Check sheet for the modelled part. Datum: model origin and axes. Units: mm. A direction names the side the tool comes from. Round coordinates to 2 decimals unless told otherwise and drop trailing zeros. Write each loop counter-clockwise with the first axis right and the second up, starting at its lowest first coordinate (ties: lowest second). Pieces come first, ordered by that corner, then holes.
Item 1: Set-up check for faces 1 (the flat face through (165.207, -94, 2)), 2 (the flat face through (83, -151, 2)), 3 (the flat face through (147, -104, 5)): record each of +Z, -Z, +X, -X, +Y, -Y from which the full face is reachable in a straight line by a thin tool's end or side.
Item 2: Section check B-B, the plane y = -133. Record the cut outline in (x, z).
Item 3: Release check for a two-part mould opening along X. For faces 4 (the flat face through (147, -104, 0)), 5 (the flat face through (172, -130.614, 2)) record: pulls with the +X half, pulls with the -X half, needs draft (parallel to the pull), parting line crosses it, or undercut.
Item 4: Section check C-C, the plane z = 2.9. State how many separate pieces and enclosed holes the cut face has, plus the area to 3 significant figures.
Item 5: Section check A-A, the plane x = 201.5. Record the cut outline in (y, z).
Item 6: Material ranges on line 1 along X through (y, z) = (-92.5, 1.2); line 2 along Y through (x, z) = (106, 4.4); line 3 along X through (y, z) = (-136.5, 3.5), recorded low to high.
Autodesk Fusion 360 part; units mm, degrees
sketch "Esquisse1" plane through (0, 0, 0) normal (0, 0, 1) x (1, 0, 0)
  line L0 (0.1341, -76.3658) -> (64.4137, -0.1129)
  line L1 (64.4137, -0.1129) -> (129.0708, -76.1647)
  line L2 (129.0708, -76.1647) -> (129.0708, -86.1624)
  line L3 (0.1341, -76.133) -> (11.9451, -86.0425)
  line L4 (129.2084, -85.9931) -> (11.8004, -85.9931)
sketch "Esquisse2" plane through (-56.9768, 0, 48.0303) normal (-0.7646, 0, 0.6445) x (0, -1, 0)
  line L0 (-20.1587, 188.3406) -> (-20.1587, 88.7874)
  line L1 (-20.1587, 88.7874) -> (127.8413, 88.7874)
  line L2 (127.8413, 88.7874) -> (127.8413, 188.3406)
  line L3 (127.8413, 188.3406) -> (-20.1587, 188.3406)
  line L4 (-18.8236, 187.8236) -> (126.1751, 187.8236)
  line L5 (126.1751, 187.8236) -> (126.1751, 87.8252)
  line L6 (126.1751, 87.8252) -> (-18.8236, 87.8252)
  line L7 (-18.8236, 87.8252) -> (-18.8236, 187.8236)
  line L8 (-3.8235, 175.0777) -> (11.1766, 175.0777)
  line L9 (11.1766, 175.0777) -> (11.1766, 160.0776)
  line L10 (11.1766, 160.0776) -> (-3.8235, 160.0776)
  line L11 (-3.8235, 160.0776) -> (-3.8235, 175.0777)
  line L12 (21.1779, 175.0777) -> (36.178, 175.0777)
  line L13 (36.178, 175.0777) -> (36.178, 160.0776)
  line L14 (36.178, 160.0776) -> (21.1779, 160.0776)
  line L15 (21.1779, 160.0776) -> (21.1779, 175.0777)
  line L16 (46.1757, 175.0777) -> (61.1758, 175.0777)
  line L17 (61.1758, 175.0777) -> (61.1758, 160.0776)
  line L18 (61.1758, 160.0776) -> (46.1757, 160.0776)
  line L19 (46.1757, 160.0776) -> (46.1757, 175.0777)
  line L20 (71.1771, 175.0777) -> (86.1772, 175.0777)
  line L21 (86.1772, 175.0777) -> (86.1772, 160.0776)
  line L22 (86.1772, 160.0776) -> (71.1771, 160.0776)
  line L23 (71.1771, 160.0776) -> (71.1771, 175.0777)
  line L24 (96.1749, 175.0777) -> (111.175, 175.0777)
  line L25 (111.175, 175.0777) -> (111.175, 160.0776)
  line L26 (111.175, 160.0776) -> (96.1749, 160.0776)
  line L27 (96.1749, 160.0776) -> (96.1749, 175.0777)
  line L28 (-3.8235, 155.1387) -> (11.1766, 155.1387)
  line L29 (11.1766, 155.1387) -> (11.1766, 140.1386)
  line L30 (11.1766, 140.1386) -> (-3.8235, 140.1386)
  line L31 (-3.8235, 140.1386) -> (-3.8235, 155.1387)
  line L32 (21.1779, 155.1387) -> (36.178, 155.1387)
  line L33 (36.178, 155.1387) -> (36.178, 140.1386)
  line L34 (36.178, 140.1386) -> (21.1779, 140.1386)
  line L35 (21.1779, 140.1386) -> (21.1779, 155.1387)
  line L36 (46.1757, 155.1387) -> (61.1758, 155.1387)
  line L37 (61.1758, 155.1387) -> (61.1758, 140.1386)
  line L38 (61.1758, 140.1386) -> (46.1757, 140.1386)
  line L39 (46.1757, 140.1386) -> (46.1757, 155.1387)
  line L40 (71.1771, 155.1387) -> (86.1772, 155.1387)
  line L41 (86.1772, 155.1387) -> (86.1772, 140.1386)
  line L42 (86.1772, 140.1386) -> (71.1771, 140.1386)
  line L43 (71.1771, 140.1386) -> (71.1771, 155.1387)
  line L44 (96.1749, 155.1387) -> (111.175, 155.1387)
  line L45 (111.175, 155.1387) -> (111.175, 140.1386)
  line L46 (111.175, 140.1386) -> (96.1749, 140.1386)
  line L47 (96.1749, 140.1386) -> (96.1749, 155.1387)
  line L48 (-3.8235, 135.1997) -> (11.1766, 135.1997)
  line L49 (11.1766, 135.1997) -> (11.1766, 120.1996)
  line L50 (11.1766, 120.1996) -> (-3.8235, 120.1996)
  line L51 (-3.8235, 120.1996) -> (-3.8235, 135.1997)
  line L52 (21.1779, 135.1997) -> (36.178, 135.1997)
  line L53 (36.178, 135.1997) -> (36.178, 120.1996)
  line L54 (36.178, 120.1996) -> (21.1779, 120.1996)
  line L55 (21.1779, 120.1996) -> (21.1779, 135.1997)
  line L56 (46.1757, 135.1997) -> (61.1758, 135.1997)
  line L57 (61.1758, 135.1997) -> (61.1758, 120.1996)
  line L58 (61.1758, 120.1996) -> (46.1757, 120.1996)
  line L59 (46.1757, 120.1996) -> (46.1757, 135.1997)
  line L60 (71.1771, 135.1997) -> (86.1772, 135.1997)
  line L61 (86.1772, 135.1997) -> (86.1772, 120.1996)
  line L62 (86.1772, 120.1996) -> (71.1771, 120.1996)
  line L63 (71.1771, 120.1996) -> (71.1771, 135.1997)
  line L64 (96.1749, 135.1997) -> (111.175, 135.1997)
  line L65 (111.175, 135.1997) -> (111.175, 120.1996)
  line L66 (111.175, 120.1996) -> (96.1749, 120.1996)
  line L67 (96.1749, 120.1996) -> (96.1749, 135.1997)
  line L68 (-3.8235, 115.2643) -> (11.1766, 115.2643)
  line L69 (11.1766, 115.2643) -> (11.1766, 100.2642)
  line L70 (11.1766, 100.2642) -> (-3.8235, 100.2642)
  line L71 (-3.8235, 100.2642) -> (-3.8235, 115.2643)
  line L72 (21.1779, 115.2643) -> (36.178, 115.2643)
  line L73 (36.178, 115.2643) -> (36.178, 100.2642)
  line L74 (36.178, 100.2642) -> (21.1779, 100.2642)
  line L75 (21.1779, 100.2642) -> (21.1779, 115.2643)
  line L76 (46.1757, 115.2643) -> (61.1758, 115.2643)
  line L77 (61.1758, 115.2643) -> (61.1758, 100.2642)
  line L78 (61.1758, 100.2642) -> (46.1757, 100.2642)
  line L79 (46.1757, 100.2642) -> (46.1757, 115.2643)
  line L80 (71.1771, 115.2643) -> (86.1772, 115.2643)
  line L81 (86.1772, 115.2643) -> (86.1772, 100.2642)
  line L82 (86.1772, 100.2642) -> (71.1771, 100.2642)
  line L83 (71.1771, 100.2642) -> (71.1771, 115.2643)
  line L84 (96.1749, 115.2643) -> (111.175, 115.2643)
  line L85 (111.175, 115.2643) -> (111.175, 100.2642)
  line L86 (111.175, 100.2642) -> (96.1749, 100.2642)
  line L87 (96.1749, 100.2642) -> (96.1749, 115.2643)
sketch "Esquisse3" plane through (0, -127.8413, 0) normal (0, -1, 0) x (1, 0, 0)
  line L0 (3.7755, 116.2201) -> (64.4218, 188.1629)
  line L1 (64.4218, 188.1629) -> (126.5708, 115.0612)
  line L2 (126.5708, 115.0612) -> (126.5708, 108.6519)
  line L3 (126.5708, 108.6519) -> (12.796, 108.6519)
  line L4 (12.796, 108.6519) -> (3.7755, 116.2201)
  line L5 (0.249, 115.9156) -> (11.8862, 106.1519)
  line L6 (11.8862, 106.1519) -> (129.0708, 106.1519)
  line L7 (129.0708, 106.1519) -> (129.0708, 115.9803)
  line L8 (129.0708, 115.9803) -> (64.4137, 192.0321)
  line L9 (64.4137, 192.0321) -> (0.249, 115.9156)
  line L10 (64.4137, 192.0321) -> (0.249, 115.9156)
  line L11 (11.8862, 106.1519) -> (129.0708, 106.1519)
  line L12 (129.0708, 115.9803) -> (64.4137, 192.0321)
sketch "Esquisse4" plane through (0, 0, 0) normal (0, 0, 1) x (1, 0, 0)
  line L0 (155.2068, -87.1605) -> (155.2068, -101.1605)
  line L1 (165.2068, -65.4335) -> (179.2068, -65.4335)
  line L2 (141.2068, -65.4335) -> (155.2068, -65.4335)
  line L3 (165.2068, -79.4335) -> (165.2068, -65.4335)
  line L4 (107.7472, -87.1605) -> (107.7472, -101.1605)
  line L5 (203.2068, -101.1605) -> (189.2068, -101.1605)
  line L6 (93.7472, -101.1605) -> (93.7472, -87.1605)
  line L7 (93.7472, -79.4335) -> (93.7472, -65.4335)
  line L8 (117.2068, -87.1605) -> (131.2068, -87.1605)
  line L9 (189.2068, -79.4335) -> (189.2068, -65.4335)
  line L10 (179.2068, -79.4335) -> (165.2068, -79.4335)
  line L11 (165.2068, -87.1605) -> (179.2068, -87.1605)
  line L12 (155.2068, -101.1605) -> (141.2068, -101.1605)
  line L13 (93.7472, -87.1605) -> (107.7472, -87.1605)
  line L14 (93.7472, -65.4335) -> (107.7472, -65.4335)
  line L15 (141.2068, -79.4335) -> (141.2068, -65.4335)
  line L16 (155.2068, -79.4335) -> (141.2068, -79.4335)
  line L17 (131.2068, -101.1605) -> (117.2068, -101.1605)
  line L18 (117.2068, -101.1605) -> (117.2068, -87.1605)
  line L19 (131.2068, -65.4335) -> (131.2068, -79.4335)
  line L20 (165.2068, -101.1605) -> (165.2068, -87.1605)
  line L21 (189.2068, -65.4335) -> (203.2068, -65.4335)
  line L22 (141.2068, -101.1605) -> (141.2068, -87.1605)
  line L23 (107.7472, -101.1605) -> (93.7472, -101.1605)
  line L24 (131.2068, -79.4335) -> (117.2068, -79.4335)
  line L25 (141.2068, -87.1605) -> (155.2068, -87.1605)
  line L26 (131.2068, -87.1605) -> (131.2068, -101.1605)
  line L27 (155.2068, -65.4335) -> (155.2068, -79.4335)
  line L28 (107.7472, -65.4335) -> (107.7472, -79.4335)
  line L29 (203.2068, -79.4335) -> (189.2068, -79.4335)
  line L30 (179.2068, -101.1605) -> (165.2068, -101.1605)
  line L31 (179.2068, -87.1605) -> (179.2068, -101.1605)
  line L32 (203.2068, -65.4335) -> (203.2068, -79.4335)
  line L33 (179.2068, -65.4335) -> (179.2068, -79.4335)
  line L34 (117.2068, -79.4335) -> (117.2068, -65.4335)
  circle A0 centre (81.9919, -61.174) radius 1.8
  line L35 (164.9366, -144.6145) -> (164.9366, -130.6145)
  line L36 (107.7472, -79.4335) -> (93.7472, -79.4335)
  line L37 (117.2068, -65.4335) -> (131.2068, -65.4335)
  line L38 (155.2068, -122.8875) -> (141.2068, -122.8875)
  line L39 (178.9366, -130.6145) -> (178.9366, -144.6145)
  line L40 (140.9366, -130.6145) -> (154.9366, -130.6145)
  circle A1 centre (81.9919, -149.174) radius 1.8
  line L41 (220.8419, -155.024) -> (75.8419, -155.024)
  line L42 (188.9366, -144.6145) -> (188.9366, -130.6145)
  line L43 (189.2068, -108.8875) -> (203.2068, -108.8875)
  line L44 (179.2068, -122.8875) -> (165.2068, -122.8875)
  line L45 (130.9366, -144.6145) -> (116.9366, -144.6145)
  line L46 (107.477, -144.6145) -> (93.477, -144.6145)
  line L47 (165.2068, -108.8875) -> (179.2068, -108.8875)
  line L48 (140.9366, -144.6145) -> (140.9366, -130.6145)
  line L49 (189.2068, -87.1605) -> (203.2068, -87.1605)
  line L50 (93.477, -144.6145) -> (93.477, -130.6145)
  line L51 (130.9366, -130.6145) -> (130.9366, -144.6145)
  line L52 (116.9366, -130.6145) -> (130.9366, -130.6145)
  line L53 (75.8419, -55.024) -> (220.8419, -55.024)
  line L54 (141.2068, -108.8875) -> (155.2068, -108.8875)
  line L55 (179.2068, -108.8875) -> (179.2068, -122.8875)
  line L56 (107.7472, -122.8875) -> (93.7472, -122.8875)
  line L57 (75.8419, -155.024) -> (75.8419, -55.024)
  line L58 (93.7472, -122.8875) -> (93.7472, -108.8875)
  line L59 (107.477, -130.6145) -> (107.477, -144.6145)
  line L60 (220.8419, -55.024) -> (220.8419, -155.024)
  line L61 (202.9366, -144.6145) -> (188.9366, -144.6145)
  line L62 (117.2068, -122.8875) -> (117.2068, -108.8875)
  line L63 (117.2068, -108.8875) -> (131.2068, -108.8875)
  line L64 (164.9366, -130.6145) -> (178.9366, -130.6145)
  line L65 (141.2068, -122.8875) -> (141.2068, -108.8875)
  line L66 (154.9366, -130.6145) -> (154.9366, -144.6145)
  line L67 (202.9366, -130.6145) -> (202.9366, -144.6145)
  circle A2 centre (214.8129, -61.174) radius 1.8
  line L68 (203.2068, -108.8875) -> (203.2068, -122.8875)
  line L69 (203.2068, -122.8875) -> (189.2068, -122.8875)
  line L70 (93.7472, -108.8875) -> (107.7472, -108.8875)
  circle A3 centre (214.8129, -149.174) radius 1.8
  line L71 (203.2068, -87.1605) -> (203.2068, -101.1605)
  line L72 (189.2068, -101.1605) -> (189.2068, -87.1605)
  line L73 (189.2068, -122.8875) -> (189.2068, -108.8875)
  line L74 (155.2068, -108.8875) -> (155.2068, -122.8875)
  line L75 (116.9366, -144.6145) -> (116.9366, -130.6145)
  line L76 (188.9366, -130.6145) -> (202.9366, -130.6145)
  line L77 (165.2068, -122.8875) -> (165.2068, -108.8875)
  line L78 (131.2068, -108.8875) -> (131.2068, -122.8875)
  line L79 (154.9366, -144.6145) -> (140.9366, -144.6145)
  line L80 (93.477, -130.6145) -> (107.477, -130.6145)
  line L81 (107.7472, -108.8875) -> (107.7472, -122.8875)
  line L82 (131.2068, -122.8875) -> (117.2068, -122.8875)
  line L83 (178.9366, -144.6145) -> (164.9366, -144.6145)
extrude "Extrusion4" add sketch "Esquisse4" along normal blind 5
hole "Perçage2" at (81.9919, -61.174, 5) direction (0, 0, -1) diameter 3.6 depth 25 tip angle 180 counterbore diameter 6.4 counterbore depth 3
hole "Perçage3" at (81.9919, -149.174, 5) direction (0, 0, -1) diameter 3.6 depth 25 tip angle 180 counterbore diameter 6.4 counterbore depth 3
hole "Perçage4" at (214.8129, -149.174, 5) direction (0, 0, -1) diameter 3.6 depth 25 tip angle 180 counterbore diameter 6.4 counterbore depth 3
hole "Perçage5" at (214.8129, -61.174, 5) direction (0, 0, -1) diameter 3.6 depth 25 tip angle 180 counterbore diameter 6.4 counterbore depth 3
Values found:
1. face 1: +Z, -Z
1. face 2: +Z
1. face 3: +Z, +X, -X, +Y, -Y
2. outline: (75.84, 0) - (93.48, 0) - (93.48, 5) - (75.84, 5) - close; (107.48, 0) - (116.94, 0) - (116.94, 5) - (107.48, 5) - close; (130.94, 0) - (140.94, 0) - (140.94, 5) - (130.94, 5) - close; (154.94, 0) - (164.94, 0) - (164.94, 5) - (154.94, 5) - close; (178.94, 0) - (188.94, 0) - (188.94, 5) - (178.94, 5) - close; (202.94, 0) - (220.84, 0) - (220.84, 5) - (202.94, 5) - close
3. face 4: needs draft
3. face 5: undercut
4. separate pieces: 1
4. enclosed holes: 24
4. area: 10,500 mm2
5. outline: (-155.02, 0) - (-144.61, 0) - (-144.61, 5) - (-155.02, 5) - close; (-130.61, 0) - (-122.89, 0) - (-122.89, 5) - (-130.61, 5) - close; (-108.89, 0) - (-101.16, 0) - (-101.16, 5) - (-108.89, 5) - close; (-87.16, 0) - (-79.43, 0) - (-79.43, 5) - (-87.16, 5) - close; (-65.43, 0) - (-55.02, 0) - (-55.02, 5) - (-65.43, 5) - close
6. line 1: x = 75.84 to 93.75, 107.75 to 117.21, 131.21 to 141.21, 155.21 to 165.21, 179.21 to 189.21, 203.21 to 220.84
6. line 2: y = -155.02 to -144.61, -130.61 to -122.89, -108.89 to -101.16, -87.16 to -79.43, -65.43 to -55.02
6. line 3: x = 75.84 to 93.48, 107.48 to 116.94, 130.94 to 140.94, 154.94 to 164.94, 178.94 to 188.94, 202.94 to 220.84
